from build123d import *

# Parameters (mm, degrees)
SKETCH1_W           = 254
SKETCH1_H           = 177.8
BOSS_EXTRUDE1_DEPTH = 12.7


with BuildPart() as part:
    # Sketch1 → Boss-Extrude1 (new body)
    with BuildSketch(Plane(origin=(0, 0, 0), x_dir=(1, 0, 0), z_dir=(0, 1, 0))):
        Rectangle(SKETCH1_W, SKETCH1_H)
    extrude(amount=BOSS_EXTRUDE1_DEPTH)

    # Cut-Sweep2: sweep along a path in Sketch2
    with BuildLine(Plane(origin=(0, 12.7, 0), x_dir=(1, 0, 0), z_dir=(0, 1, 0))) as cut_sweep2_path:
        Line((20.796437491, -88.9), (20.796437491, -47.488713932))
        ThreePointArc((20.796437491, -47.488713932), (14.100898509, -31.324252914), (-2.063562509, -24.628713932))
        Line((-2.063562509, -24.628713932), (-27.110242968, -24.628713932))
        Line((-27.110242968, -24.628713932), (-43.640180234, -24.628713932))
        ThreePointArc((-43.640180234, -24.628713932), (-59.804641252, -17.93317495), (-66.500180234, -1.768713932))
        Line((-66.500180234, -1.768713932), (-66.500180234, 0.806968371))
        ThreePointArc((-66.500180234, 0.806968371), (-59.804641252, 16.971429389), (-43.640180234, 23.666968371))
        Line((-43.640180234, 23.666968371), (30.223833761, 23.666968371))
        ThreePointArc((30.223833761, 23.666968371), (48.184346003, 16.227480613), (55.623833761, -1.733031629))
        Line((55.623833761, -1.733031629), (55.623833761, -43.941009117))
        ThreePointArc((55.623833761, -43.941009117), (60.831475192, -56.513367686), (73.403833761, -61.721009117))
        Line((73.403833761, -61.721009117), (74.093236775, -61.721009117))
        ThreePointArc((74.093236775, -61.721009117), (86.665595344, -56.513367686), (91.873236775, -43.941009117))
        Line((91.873236775, -43.941009117), (91.873236775, 26.14139739))
        ThreePointArc((91.873236775, 26.14139739), (80.714005138, 53.082165753), (53.773236775, 64.24139739))
        Line((53.773236775, 64.24139739), (-65.356762302, 64.24139739))
        ThreePointArc((-65.356762302, 64.24139739), (-92.297530666, 53.082165753), (-103.456762302, 26.14139739))
        Line((-103.456762302, 26.14139739), (-103.456762302, -24.595886827))
        ThreePointArc((-103.456762302, -24.595886827), (-92.297530666, -51.53665519), (-65.356762302, -62.695886827))
        Line((-65.356762302, -62.695886827), (-43.57480307, -62.695886827))
        ThreePointArc((-43.57480307, -62.695886827), (-30.104418888, -68.275502645), (-24.52480307, -81.745886827))
        Line((-24.52480307, -81.745886827), (-24.52480307, -88.9))
    # Sketch3 → Cut-Sweep2 (sweep, cut)
    with BuildSketch(Plane.XY.offset(88.9)):
        with BuildLine():
            Line((-16.90480307, 12.7), (-16.90480307, 9.380942321))
            ThreePointArc((-16.90480307, 9.380942321), (-24.52480307, 1.760942321), (-32.14480307, 9.380942321))
            Line((-32.14480307, 9.380942321), (-32.14480307, 12.7))
            ThreePointArc((-32.14480307, 12.7), (-24.52480307, 20.32), (-16.90480307, 12.7))
        make_face()
    sweep(path=cut_sweep2_path.line, mode=Mode.SUBTRACT)


solid = part.part
Here's how the part is built. I have some questions about the finished solid (model axes, mm). A direction names the side the tool comes from. Coordinates: 2 decimals unless noted, no trailing zeros.
1) Thinking about a two-plate mould opening in Z: for faces 1 (the face through (-2, 6, 88.9)), 2 (the face through (127, 6, 1)), 3 (the face through (8.8, 11.1, 36.8)), which applies, +Z half, -Z half, draft (parallel to the pull), parting line (faces both ways), or undercut?
Filled in:
face 1: +Z half
face 2: draft
face 3: undercut
2) If I drill on line 1 (X direction, y = 6.5, z = 23.5); line 2 (Z direction, x = 78.5, y = 3.25); line 3 (Z direction, x = -10, y = 7.25), over which ranges is the centre line in solid material (lowest first)?
Filled in:
line 1: x = -127 to -110.51, -96.4 to -64.2, 15.81 to 48.57, 62.68 to 84.82, 98.93 to 127
line 2: z = -88.9 to -60.86, -48.85 to 56.44, 65.81 to 88.9
line 3: z = -88.9 to -71.56, -56.93 to -30.98, -16.35 to 17.31, 31.94 to 88.9
3) Which directions (+Z, -Z, +X, -X, +Y, -Y) give clear straight access to the entire face, cutting with the end or side of a thin tool? Please do faces 4 (the face through (-2, 12.7, -1)), 5 (the face through (-24.692, 1.763, 85.373)), 6 (the face through (-35.582, 11.017, 73.575)).
Filled in:
face 4: +Z, -Z, +X, -X, +Y
face 5: +Z, +Y
face 6: +Y
